Answer from the drawing. Dimensions are ordinates in mm from the lowest x, y and z of the part. A direction names the side the tool comes from. Round coordinates to 2 decimals unless told otherwise and drop trailing zeros. Loops run counter-clockwise (first coordinate to the right, second up) from the corner with the lowest first, then second, coordinate; pieces in that order, holes last. Notation, with made-up numbers: (19.5, 67) - (42.5, 67) arc R25 cw to (42.5, 88) - close; hole circle Ø8 at (19, 65). An arc over 180 degrees is marked (long way). Answer as CSV lines item,"result". Start each with the question number.
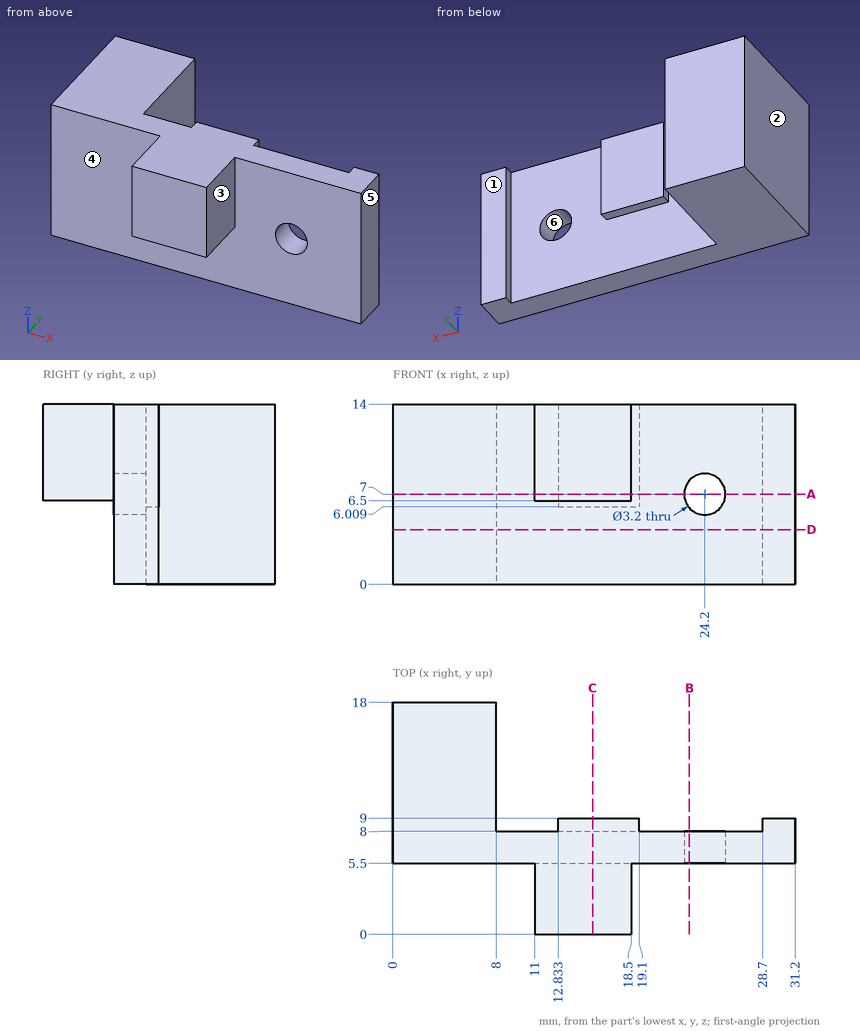
Item 1: Section D-D, the plane z = 4.25 is taken. Give the vertices of the cut face in (x, y).
Item 2: Find the intervals of material crossed by L1, parallel to Z at x = 24.2, y = 7.15; L2, parallel to X at y = 6.1, z = 7; L3, parallel to Y at x = 17.5, z = 10.25, in increasing order.
Item 3: Flat-ended cylindrical pins translate along their axes: pin 1 Ø1.9 at (x, z) = (24.2, 7) entering from +Y; pin 2 Ø2 at (x, z) = (30, 7.5) entering from +Y; pin 3 Ø5 at (x, y) = (10.5, 2.5) entering from -Z; pin 4 Ø1.5 at (y, z) = (3, 9.5) entering from -X. Find the tip coordinate at first contact, or state that the pin passes through.
Item 4: Section C-C, the plane x = 15.5 is taken. Give the vertices of the cut face in (y, z).
Item 5: Section B-B, the plane x = 23 is taken. Give the vertices of the cut face in (y, z), and give its area (3 significant figures).
Item 6: Section A-A, the plane z = 7 is taken. Give the vertices of the cut face in (x, y), and give its area (3 significant figures).
Item 7: Which of the six approach directions +Z, -Z, +X, -X, +Y, -Y give full straight-line access (tool end or side, diameter ignored) to the marked faces 1, 2 and 3?
Item 8: Determine the mould class of the marked faces 4, 5 and 6 for opening direction X: pulls with the +X half, pulls with the -X half, needs draft (parallel to the pull), parting line crosses it, or undercut.
Answer:
1,outline,"(0, 5.5) - (31.2, 5.5) - (31.2, 9) - (28.7, 9) - (28.7, 8) - (8, 8) - (8, 18) - (0, 18) - close"
2,L1,"z = 0 to 5.4, 8.6 to 14"
2,L2,"x = 0 to 22.6, 25.8 to 31.2"
2,L3,"y = 0 to 9"
3,pin 1,"passes through"
3,pin 2,"stops at y = 9"
3,pin 3,"stops at z = 6.5"
3,pin 4,"stops at x = 11"
4,outline,"(0, 6.5) - (5.5, 6.5) - (5.5, 0) - (8, 0) - (8, 6.01) - (9, 6.01) - (9, 14) - (0, 14) - close"
5,outline,"(5.5, 0) - (8, 0) - (8, 5.94) - (5.5, 5.94) - close; (5.5, 8.06) - (8, 8.06) - (8, 14) - (5.5, 14) - close"
5,area,"29.7 mm²"
6,outline,"(0, 5.5) - (11, 5.5) - (11, 0) - (18.5, 0) - (18.5, 5.5) - (22.6, 5.5) - (22.6, 8) - (19.1, 8) - (19.1, 9) - (12.83, 9) - (12.83, 8) - (8, 8) - (8, 18) - (0, 18) - close; (25.8, 5.5) - (31.2, 5.5) - (31.2, 9) - (28.7, 9) - (28.7, 8) - (25.8, 8) - close"
6,area,"200 mm²"
7,face 1,"+Z, -Z, +X, +Y"
7,face 2,"+Z, -Z, -X, +Y, -Y"
7,face 3,"+Z, -Z, +X, -Y"
8,face 4,"needs draft"
8,face 5,"pulls with the +X half"
8,face 6,"undercut"
